The listing builds one solid part. Answer for the finished solid, in the listing's coordinates (mm). Give positions to 0.01 mm unless a question says otherwise; leave off trailing zeros. Order: outer loops, then holes, each group sorted by start corner. A loop starts at its lowest first (then second) coordinate and runs counter-clockwise, first axis right, second up. Notation, with made-up numbers: M 64,57 L 74,57 A3 cw 74,62 Z; hole C -36.5,16 d8. An arc over 180 degrees is marked long. Answer as a JSON object with one key per item and string values. Group by question number.
```python
from build123d import *

# Parameters (mm, degrees)
F0_W         = 135.5529725552
F0_H         = 64.4017234445
F1_DEPTH     = 8
F2_R         = 5
F3_T1_DEPTH  = 25.5
F3_T4_ANGLE  = 90
F3_T6_ANGLE  = 90
F3_T8_ANGLE  = 90
F3_T10_ANGLE = 90
F4_R         = 1
F5_W         = 105.8298870921
F5_H         = 54.4540472329
F6_DEPTH     = 1


# Not quite as in the source:
# - a fillet or chamfer that OpenCascade refuses, or shapes differently, is made with other operations: its cross-section is extruded or revolved along the edge and cut away or added


with BuildPart() as f1:
    # F0 (on Top) → F1 (new body)
    with BuildSketch(Plane.XY):
        Rectangle(F0_W, F0_H)
    extrude(amount=F1_DEPTH)

    # F2
    f2_edges = [f1.edges().sort_by_distance(p)[0] for p in [
        (0, 32.200862, 8),
        (-67.776486, 0, 8),
        (0, -32.200862, 8),
        (67.776486, 0, 8),
    ]]
    fillet(f2_edges, radius=F2_R)

    # F3: fillet of radius 7 on 4 edges, made by hand

    # F3_s2 → F3_t1 (cut)
    with BuildSketch(Plane.XY.offset(-17.5)):
        with BuildLine():
            ThreePointArc((-67.7764862776, -25.2008617222), (-65.7262337459, -30.1506091905), (-60.7764862776, -32.2008617222))
            Line((-60.7764862776, -32.2008617222), (-67.7764862776, -32.2008617222))
            Line((-67.7764862776, -32.2008617222), (-67.7764862776, -25.2008617222))
        make_face()
        with BuildLine():
            ThreePointArc((60.7764862776, -32.2008617222), (65.7262337459, -30.1506091905), (67.7764862776, -25.2008617222))
            Line((67.7764862776, -25.2008617222), (67.7764862776, -32.2008617222))
            Line((67.7764862776, -32.2008617222), (60.7764862776, -32.2008617222))
        make_face()
        with BuildLine():
            ThreePointArc((60.7764862776, 32.2008617222), (65.7262337459, 30.1506091905), (67.7764862776, 25.2008617222))
            Line((67.7764862776, 25.2008617222), (67.7764862776, 32.2008617222))
            Line((67.7764862776, 32.2008617222), (60.7764862776, 32.2008617222))
        make_face()
        with BuildLine():
            ThreePointArc((-67.7764862776, 25.2008617222), (-65.7262337459, 30.1506091905), (-60.7764862776, 32.2008617222))
            Line((-60.7764862776, 32.2008617222), (-67.7764862776, 32.2008617222))
            Line((-67.7764862776, 32.2008617222), (-67.7764862776, 25.2008617222))
        make_face()
    extrude(amount=F3_T1_DEPTH, mode=Mode.SUBTRACT)

    # F3_s3 → F3_t4 (revolve, cut)
    with BuildSketch(Plane.YZ.offset(-60.7764862776)):
        with BuildLine():
            ThreePointArc((27.2008617222, 8), (30.7363956282, 6.5355339059), (32.2008617222, 3))
            Line((32.2008617222, 3), (32.2008617222, 8))
            Line((32.2008617222, 8), (27.2008617222, 8))
        make_face()
    revolve(axis=Axis((-60.7764862776, 25.2008617222, 8), (0, 0, 1)), revolution_arc=F3_T4_ANGLE, mode=Mode.SUBTRACT)

    # F3_s5 → F3_t6 (revolve, cut)
    with BuildSketch(Plane.XZ.offset(-25.2008617222)):
        with BuildLine():
            ThreePointArc((62.7764862776, 8), (66.3120201835, 6.5355339059), (67.7764862776, 3))
            Line((67.7764862776, 3), (67.7764862776, 8))
            Line((67.7764862776, 8), (62.7764862776, 8))
        make_face()
    revolve(axis=Axis((60.7764862776, 25.2008617222, 8), (0, 0, 1)), revolution_arc=F3_T6_ANGLE, mode=Mode.SUBTRACT)

    # F3_s7 → F3_t8 (revolve, cut)
    with BuildSketch(Plane.YZ.offset(60.7764862776)):
        with BuildLine():
            ThreePointArc((-27.2008617222, 8), (-30.7363956282, 6.5355339059), (-32.2008617222, 3))
            Line((-32.2008617222, 3), (-32.2008617222, 8))
            Line((-32.2008617222, 8), (-27.2008617222, 8))
        make_face()
    revolve(axis=Axis((60.7764862776, -25.2008617222, 8), (0, 0, 1)), revolution_arc=F3_T8_ANGLE, mode=Mode.SUBTRACT)

    # F3_s9 → F3_t10 (revolve, cut)
    with BuildSketch(Plane.XZ.offset(25.2008617222)):
        with BuildLine():
            ThreePointArc((-62.7764862776, 8), (-66.3120201835, 6.5355339059), (-67.7764862776, 3))
            Line((-67.7764862776, 3), (-67.7764862776, 8))
            Line((-67.7764862776, 8), (-62.7764862776, 8))
        make_face()
    revolve(axis=Axis((-60.7764862776, -25.2008617222, 8), (0, 0, 1)), revolution_arc=F3_T10_ANGLE, mode=Mode.SUBTRACT)

    # F4
    f4_edges = [f1.edges().sort_by_distance(p)[0] for p in [
        (0, -32.200862, 0),
        (-67.776486, 0, 0),
    ]]
    fillet(f4_edges, radius=F4_R)

    # F5 (on face) → F6 (cut)
    with BuildSketch(Plane(origin=(0, 0, 0), x_dir=(1, 0, 0), z_dir=(0, 0, -1))):
        Rectangle(F5_W, F5_H)
    extrude(amount=-F6_DEPTH, mode=Mode.SUBTRACT)


solid = f1.part
```
Item 1: Flat-ended cylindrical pins translate along their axes: P1, Ø0.8, axis at y = 3.5, z = 0.5, coming from the +X side; P2, Ø8, axis at x = -11.5, y = -11.5, coming from the -Z side; P3, Ø0.8, axis at x = -16.5, z = 0.5, coming from the -Y side; P4, Ø1.1, axis at y = 0, z = 0.5, coming from the -X side. Find the tip coordinate at first contact, or state that the pin passes through.
Item 2: Section A-A (y = 4) is taken. Determine the outline of the cut face in (x, z).
Item 3: Section B-B (x = -35) is taken. Determine the outline of the cut face in (y, z), and give its area (3 significant figures).
Item 4: Determine the mould class of faces 1 (the flat face through (-1, 0, 1)), 2 (the cylindrical face through (-66.35, 0.35, 6.5)), 3 (the cylindrical face through (0.851, 30.775, 6.496)) for opening direction X: released by +X, released by -X, zero draft, split by the parting line, or undercut.
Item 5: Consider probe 1 along Z at (x, y) = (-3.5, 14); probe 2 along X at (y, z) = (-19.5, 0.75); probe 3 along X at (y, z) = (-4, 0.5). Determine where each line is inside the solid, lowest interval first. Write a range as from..to.
Values found:
{
 "1": {"P1": "stops at x = 67.77", "P2": "stops at z = 1", "P3": "stops at y = -32.2", "P4": "stops at x = -67.78"},
 "2": {"outline": "M -67.78,1 A1 ccw -66.78,0 L -52.91,0 L -52.91,1 L 52.91,1 L 52.91,0 L 66.78,0 A1 ccw 67.78,1 L 67.78,3 A5 ccw 62.78,8 L -62.78,8 A5 ccw -67.78,3 Z"},
 "3": {"outline": "M -32.2,1 A1 ccw -31.2,0 L -27.23,0 L -27.23,1 L 27.23,1 L 27.23,0 L 31.2,0 A1 ccw 32.2,1 L 32.2,3 A5 ccw 27.2,8 L -27.2,8 A5 ccw -32.2,3 Z", "area": "450 mm^2"},
 "4": {"face 1": "undercut", "face 2": "released by -X", "face 3": "zero draft"},
 "5": {"probe 1": "z = 1..8", "probe 2": "x = -67.74..-52.91, 52.91..67.74", "probe 3": "x = -67.64..-52.91, 52.91..67.64"}
}
